Here's how the part is built. I have some questions about the finished solid (model axes, mm). A direction names the side the tool comes from. Give positions to 0.01 mm unless a question says otherwise; leave off trailing zeros. Write each loop counter-clockwise with the first axis right and the second up, starting at its lowest first coordinate (ties: lowest second). Pieces come first, ordered by that corner, then holes. Notation, with made-up numbers: (11, 2.25) - (25, 2.25) arc R11 cw to (25, 22.25) - close; hole circle Ø8 at (26, 39.25). An arc over 180 degrees is marked (long way). Use a Markdown table: item, result.
```python
from build123d import *

# Parameters (mm, degrees)
BOSS_EXTRUDE5_DEPTH      = 18
BOSS_EXTRUDE6_DEPTH      = 14.5
BOSS_EXTRUDE6_DEPTH_BACK = 32.5
SKETCH5_R                = 72
SKETCH5_R_2              = 61


with BuildPart() as part:
    # Sketch1 → Boss-Extrude5 (new body)
    with BuildSketch(Plane.XY):
        with BuildLine():
            ThreePointArc((-30.757316719, -52.678149818), (-10.195342734, -60.141956956), (11.677704627, -59.871789807))
            ThreePointArc((11.677704627, -59.871789807), (8.429841492, -58.288205935), (9.060512734, -54.730312371))
            ThreePointArc((9.060512734, -54.730312371), (19.779749173, -36.530020554), (18.79448635, -15.430686222))
            ThreePointArc((18.79448635, -15.430686222), (17.483891441, -9.285507816), (17.746946993, -3.007635689))
            ThreePointArc((17.746946993, -3.007635689), (17.99859257, -0.225089943), (17.816611705, 2.562878725))
            ThreePointArc((17.816611705, 2.562878725), (19.790690206, 9.581605585), (26.315634879, 12.835005296))
            ThreePointArc((26.315634879, 12.835005296), (52.449565984, -1.128017494), (52.67814252, -30.757329218))
            ThreePointArc((52.67814252, -30.757329218), (60.141955689, -10.195350207), (59.871789938, 11.677703954))
            ThreePointArc((59.871789938, 11.677703954), (58.288206152, 8.429840898), (54.730312659, 9.060511918))
            ThreePointArc((54.730312659, 9.060511918), (36.530019461, 19.779748115), (15.430684033, 18.794485892))
            ThreePointArc((15.430684033, 18.794485892), (9.285506382, 17.48389147), (3.007635099, 17.746947093))
            ThreePointArc((3.007635099, 17.746947093), (0.225087357, 17.998592603), (-2.562883253, 17.816611054))
            ThreePointArc((-2.562883253, 17.816611054), (-9.581612202, 19.790686823), (-12.835014333, 26.315631712))
            ThreePointArc((-12.835014333, 26.315631712), (1.128002953, 52.449566526), (30.757315296, 52.678150649))
            ThreePointArc((30.757315296, 52.678150649), (10.195341286, 60.141957202), (-11.677705893, 59.87178956))
            ThreePointArc((-11.677705893, 59.87178956), (-8.429842727, 58.288205762), (-9.060513882, 54.730312188))
            ThreePointArc((-9.060513882, 54.730312188), (-19.779749829, 36.530020233), (-18.794486597, 15.430686052))
            ThreePointArc((-18.794486597, 15.430686052), (-17.48389156, 9.285507447), (-17.746947093, 3.007635099))
            ThreePointArc((-17.746947093, 3.007635099), (-17.998592591, 0.225088317), (-17.816611327, -2.56288135))
            ThreePointArc((-17.816611327, -2.56288135), (-19.790686113, -9.581611967), (-26.315632103, -12.835014885))
            ThreePointArc((-26.315632103, -12.835014885), (-52.44956681, 1.128003994), (-52.678149652, 30.757317003))
            ThreePointArc((-52.678149652, 30.757317003), (-60.141956871, 10.195343235), (-59.871789938, -11.677703952))
            ThreePointArc((-59.871789938, -11.677703952), (-58.288206008, -8.429840823), (-54.73031244, -9.060512152))
            ThreePointArc((-54.73031244, -9.060512152), (-36.530020387, -19.779749225), (-15.430685526, -18.794486492))
            ThreePointArc((-15.430685526, -18.794486492), (-9.285507097, -17.483891569), (-3.007634946, -17.746947119))
            ThreePointArc((-3.007634946, -17.746947119), (-0.225087887, -17.998592596), (2.562882049, -17.816611227))
            ThreePointArc((2.562882049, -17.816611227), (9.581611647, -19.79068664), (12.835014058, -26.315631978))
            ThreePointArc((12.835014058, -26.315631978), (-1.128004083, -52.449566659), (-30.757316719, -52.678149818))
        make_face()
    extrude(amount=-BOSS_EXTRUDE5_DEPTH)

    # Sketch5 → Boss-Extrude6 (add, two sides: drawn at the far end of the back side and taken through both)
    with BuildSketch(Plane.XY.offset(-BOSS_EXTRUDE6_DEPTH_BACK)):
        Circle(SKETCH5_R)
        Circle(SKETCH5_R_2, mode=Mode.SUBTRACT)
    extrude(amount=BOSS_EXTRUDE6_DEPTH + BOSS_EXTRUDE6_DEPTH_BACK)


solid = part.part
```
Item 1: If we section it at B-B, the plane z = -6.5: Count the separate pieces of the cut face and the enclosed holes in it, plus the area to 3 significant figures.
Values:
| item | result |
|---|---|
| separate pieces | 1 |
| enclosed holes | 4 |
| area | 7,830 mm2 |
Item 2: Will these pins go through, and if not, where does the flat tip stop? pin 1 Ø1.5 at (x, y) = (17.5, -16) entering from +Z; pin 2 Ø5 at (y, z) = (-31, -3) entering from +X; pin 3 Ø2 at (x, z) = (34.5, -14) entering from -Y.
Values:
| item | result |
|---|---|
| pin 1 | stops at z = 0 |
| pin 2 | stops at x = 66.12 |
| pin 3 | stops at y = -63.73 |
Item 3: I need wall thicknesses on line 1 along Y through (x, z) = (0, -13); line 2 along Y through (x, z) = (47.5, -2); line 3 along X through (y, z) = (-54, -12). Which ranges of each line are inside material? Lowest first, please. Write a range as [from, to].
Values:
| item | result |
|---|---|
| line 1 | y = [-72, -51.73], [-18, 18], [51.73, 72] |
| line 2 | y = [-54.11, -38.27], [4.99, 15.08], [38.27, 54.11] |
| line 3 | x = [-47.62, -28.21], [-4.06, 9.82], [28.37, 47.62] |
Item 4: If we section it at A-A, the plane x = 0: Write out the boundary of the cut face in (y, z).
Values:
| item | result |
|---|---|
| outline | (-72, -32.5) - (-61, -32.5) - (-61, -18) - (-51.73, -18) - (-51.73, 0) - (-61, 0) - (-61, 14.5) - (-72, 14.5) - close; (-18, -18) - (18, -18) - (18, 0) - (-18, 0) - close; (51.73, -18) - (61, -18) - (61, -32.5) - (72, -32.5) - (72, 14.5) - (61, 14.5) - (61, 0) - (51.73, 0) - close |
Item 5: If we section it at D-D, the plane z = 5: Write out the boundary of the cut face in (x, y), plus the area to 3 significant figures.
Values:
| item | result |
|---|---|
| outline | circle Ø144 at (0, 0); hole circle Ø122 at (0, 0) |
| area | 4,600 mm2 |
Item 6: Thinking about a two-plate mould opening in Y: for faces 1 (the cylindrical face through (0, -18, -9)), 2 (the flat face through (0, 0, -18)), 3 (the flat face through (-59, 16.3, -32.5)), which applies, +Y half, -Y half, draft (parallel to the pull), parting line (faces both ways), or undercut?
Values:
| item | result |
|---|---|
| face 1 | undercut |
| face 2 | undercut |
| face 3 | draft |
Item 7: For faces 4 (the cylindrical face through (58.183, 18.323, -9.329)), 5 (the cylindrical face through (17.49, -9.37, -8.87)), which set-ups out of +Z, -Z, +X, -X, +Y, -Y let a thin tool reach every point of the face, with its end or its side?
Values:
| item | result |
|---|---|
| face 4 | none |
| face 5 | +Z, -Z |
